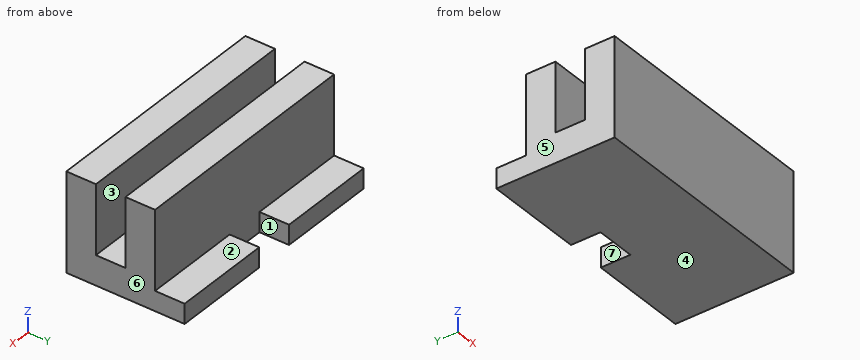
```python
from build123d import *

# Parameters (mm, degrees)
SKETCH1_W           = 12
SKETCH1_H           = 5
BOSS_EXTRUDE1_DEPTH = 4.5
CUT_EXTRUDE1_START  = -1.5
SKETCH2_W           = 12
SKETCH2_H           = 3.5
CUT_EXTRUDE1_DEPTH  = 1.5
SKETCH4_W           = 5
SKETCH4_H           = 1
BOSS_EXTRUDE2_DEPTH = 1.5


with BuildPart() as part:
    # Sketch1 → Boss-Extrude1 (new body)
    with BuildSketch(Plane(origin=(0, 0, 0), x_dir=(1, 0, 0), z_dir=(0, 1, 0))):
        with Locations((6, -2.5)):
            Rectangle(SKETCH1_W, SKETCH1_H)
    extrude(amount=BOSS_EXTRUDE1_DEPTH)

    # Sketch2 → Cut-Extrude1 (cut)
    with BuildSketch(Plane(origin=(0, 4.5, 0), x_dir=(1, 0, 0), z_dir=(0, 1, 0)).offset(CUT_EXTRUDE1_START)):
        with Locations((6, -3.25)):
            Rectangle(SKETCH2_W, SKETCH2_H)
    extrude(amount=-CUT_EXTRUDE1_DEPTH, mode=Mode.SUBTRACT)

    # Sketch4 → Boss-Extrude2 (add)
    with BuildSketch(Plane(origin=(0, 4.5, 0), x_dir=(1, 0, 0), z_dir=(0, 1, 0))):
        with Locations((2.5, -0.5)):
            Rectangle(SKETCH4_W, SKETCH4_H)
        with Locations((9.5, -0.5)):
            Rectangle(SKETCH4_W, SKETCH4_H)
    extrude(amount=BOSS_EXTRUDE2_DEPTH)


solid = part.part
```
The model under review builds one solid part; all positions refer to its coordinate system, in mm. Face numbers are marked on the shaded views. A direction names the side the tool comes from. Coordinates: 2 decimals unless noted, no trailing zeros. Order: outer loops, then holes, each group sorted by start corner. A loop starts at its lowest first (then second) coordinate and runs counter-clockwise, first axis right, second up. Notation, with made-up numbers: (-17, 62) -> (28, 62) arc R20 cw to (28, 94) -> close; hole circle Ø5 at (-24, 52.25). An arc over 180 degrees is marked (long way). Answer in a Markdown table with one row per item. Add a question column.
Item 1: We need section B-B on x = 9. Write out the cut boundary in (y, z).
Item 2: Clearance check with a flat-ended pin moving along its axis: pin 1 (1 mm diameter, centred on x = 8.5, z = 3, fed in from +Y). State where the tip first meets the part, or that it passes through.
Item 3: We need section C-C on z = 3.85. Write out the cut boundary in (x, y), plus the area to 3 significant figures.
Item 4: We need section D-D on z = 0.75. Write out the cut boundary in (x, y), plus the area to 3 significant figures.
Item 5: We need section A-A on y = 5.55. Write out the cut boundary in (x, z).
Item 6: To check wall thickness, follow probe 1 along Y at (x, z) = (10, 3.2); probe 2 along X at (y, z) = (5.65, 0.55); probe 3 along Z at (x, y) = (7.5, 4.65). State the ranges of each line that lie inside material, in increasing order.
Item 7: Mouldability with a two-part tool opening along X and no side actions: class the marked faces 4, 5, 6 and 7 as +X half, -X half, draft (parallel to the pull), parting line (faces both ways), or undercut.
Item 8: Machinability: for the marked faces 1, 2 and 3, which of the approach directions +Z, -Z, +X, -X, +Y, -Y give a long, thin tool a straight path to every point of the face, cutting with its end or side? Answer none if there is none.
Final values:
| question | item | result |
|---|---|---|
| 1 | outline | (0, 0) -> (6, 0) -> (6, 1) -> (4.5, 1) -> (4.5, 5) -> (3, 5) -> (3, 1.5) -> (1.5, 1.5) -> (1.5, 5) -> (0, 5) -> close |
| 2 | pin 1 | stops at y = 4.5 |
| 3 | outline | (0, 0) -> (12, 0) -> (12, 1.5) -> (0, 1.5) -> close; (0, 3) -> (12, 3) -> (12, 4.5) -> (0, 4.5) -> close |
| 3 | area | 36.0 mm2 |
| 4 | outline | (0, 0) -> (12, 0) -> (12, 6) -> (7, 6) -> (7, 4.5) -> (5, 4.5) -> (5, 6) -> (0, 6) -> close |
| 4 | area | 69.0 mm2 |
| 5 | outline | (0, 0) -> (5, 0) -> (5, 1) -> (0, 1) -> close; (7, 0) -> (12, 0) -> (12, 1) -> (7, 1) -> close |
| 6 | probe 1 | y = 0 to 1.5, 3 to 4.5 |
| 6 | probe 2 | x = 0 to 5, 7 to 12 |
| 6 | probe 3 | z = 0 to 1 |
| 7 | face 4 | draft |
| 7 | face 5 | -X half |
| 7 | face 6 | +X half |
| 7 | face 7 | undercut |
| 8 | face 1 | +Z, -Z, +Y |
| 8 | face 2 | +Z, +X, -X, +Y |
| 8 | face 3 | +Z, +X, -X |
